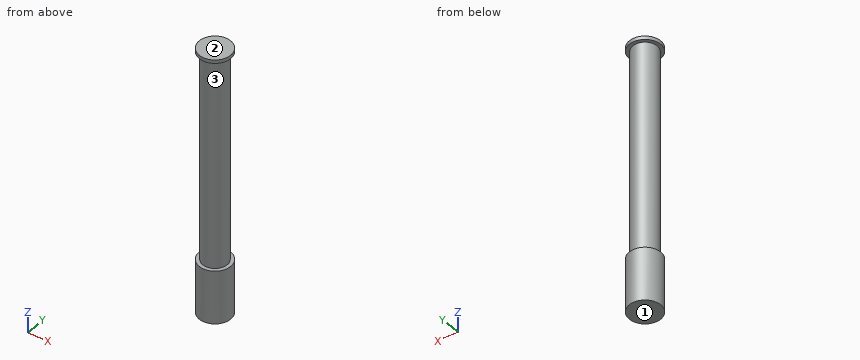
from build123d import *

# Parameters (mm, degrees)
SKETCH1_R           = 2.25
BOSS_EXTRUDE1_DEPTH = 38.1
CUT_EXTRUDE1_START  = -7.62
SKETCH3_OUTSIDE_W   = 14.226
SKETCH3_OUTSIDE_H   = 14.226
SKETCH3_OUTSIDE_R   = 1.75
CUT_EXTRUDE1_DEPTH  = 29.98


with BuildPart() as part:
    # Sketch1 → Boss-Extrude1 (new body)
    with BuildSketch(Plane.XY):
        with Locations(Location((0, 5.826393973, 0), (0, 0, 180))):
            Circle(SKETCH1_R)
    extrude(amount=BOSS_EXTRUDE1_DEPTH)

    # Sketch3 outside → Cut-Extrude1 (cut)
    with BuildSketch(Plane(origin=(0, 0, 0), x_dir=(-1, 0, 0), z_dir=(0, 0, -1)).offset(CUT_EXTRUDE1_START)):
        with Locations((0, 5.826)):
            Rectangle(SKETCH3_OUTSIDE_W, SKETCH3_OUTSIDE_H)
        with Locations((0, 5.826393973)):
            Circle(SKETCH3_OUTSIDE_R, mode=Mode.SUBTRACT)
    extrude(amount=-CUT_EXTRUDE1_DEPTH, mode=Mode.SUBTRACT)


solid = part.part
Input: part model. Units: mm. Frame: model coordinates. Face numbers are marked on the shaded views. Round coordinates to 2 decimals unless told otherwise and drop trailing zeros. Write each loop counter-clockwise with the first axis right and the second up, starting at its lowest first coordinate (ties: lowest second). Pieces come first, ordered by that corner, then holes.
1) Ray query, L1, parallel to Z at x = -1.8, y = 5.55; L2, parallel to Y at x = -0.1, z = 10; L3, parallel to X at y = 5.7, z = 26. Return the intervals inside material, ascending.
2) Draft query along Z for the marked faces 1, 2 and 3. Return one class per face: pulls with the +Z half, pulls with the -Z half, needs draft (parallel to the pull), parting line crosses it, or undercut.
3) Cut plane C-C (z = 16.5). Return the cut outline in (x, y).
4) Contact query for flat-ended pins moving along their axis: P1, Ø1, axis at x = 0, z = 22.5, coming from the -Y side; P2, Ø2, axis at x = -0.5, z = 17.5, coming from the +Y side. Output: stop coordinate, or through.
5) Cut plane A-A (x = 0). Return the cut outline in (y, z).
6) Cut plane B-B (y = 5.2). Return the cut outline in (x, z).
Geometry says:
1. L1: z = 0 to 7.62, 37.6 to 38.1
1. L2: y = 4.08 to 7.57
1. L3: x = -1.75 to 1.75
2. face 1: pulls with the -Z half
2. face 2: pulls with the +Z half
2. face 3: undercut
3. outline: circle Ø3.5 at (0, 5.83)
4. P1: stops at y = 4.08
4. P2: stops at y = 7.58
5. outline: (3.58, 0) - (8.08, 0) - (8.08, 7.62) - (7.58, 7.62) - (7.58, 37.6) - (8.08, 37.6) - (8.08, 38.1) - (3.58, 38.1) - (3.58, 37.6) - (4.08, 37.6) - (4.08, 7.62) - (3.58, 7.62) - close
6. outline: (-2.16, 0) - (2.16, 0) - (2.16, 7.62) - (1.63, 7.62) - (1.63, 37.6) - (2.16, 37.6) - (2.16, 38.1) - (-2.16, 38.1) - (-2.16, 37.6) - (-1.63, 37.6) - (-1.63, 7.62) - (-2.16, 7.62) - close
